```python
from build123d import *

# Parameters (mm, degrees)
SKETCH1_R           = 35
BOSS_EXTRUDE2_DEPTH = 10
SKETCH2_R           = 31
CUT_EXTRUDE1_DEPTH  = 5
SKETCH3_R           = 1.5
BOSS_EXTRUDE3_DEPTH = 5


with BuildPart() as part:
    # Sketch1 → Boss-Extrude2 (new body)
    with BuildSketch(Plane(origin=(0, 0, 0), x_dir=(1, 0, 0), z_dir=(0, 1, 0))):
        Circle(SKETCH1_R)
    extrude(amount=BOSS_EXTRUDE2_DEPTH)

    # Sketch2 → Cut-Extrude1 (cut)
    with BuildSketch(Plane(origin=(0, 10, 0), x_dir=(1, 0, 0), z_dir=(0, 1, 0))):
        Circle(SKETCH2_R)
    extrude(amount=-CUT_EXTRUDE1_DEPTH, mode=Mode.SUBTRACT)

    # Sketch3 → Boss-Extrude3 (add)
    with BuildSketch(Plane.XZ):
        Circle(SKETCH3_R)
    extrude(amount=BOSS_EXTRUDE3_DEPTH)


solid = part.part
```
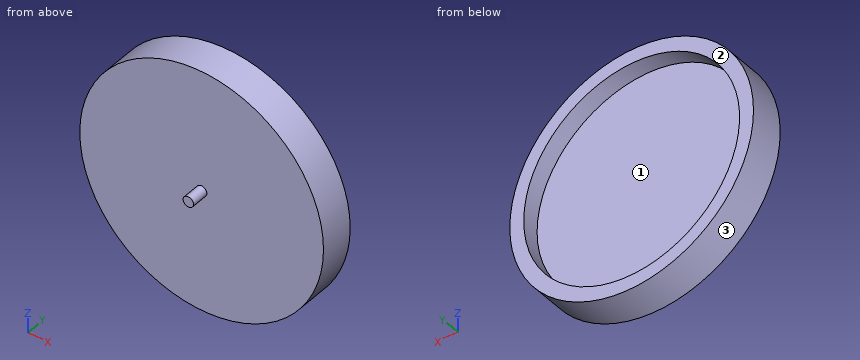
Model file for the job. Use its own axes, mm. Face numbers are marked on the shaded views. Round coordinates to 2 decimals unless told otherwise and drop trailing zeros. Write each loop counter-clockwise with the first axis right and the second up, starting at its lowest first coordinate (ties: lowest second). Pieces come first, ordered by that corner, then holes. Notation, with made-up numbers: (48.5, -24.5) - (67.5, -24.5) arc R19 cw to (67.5, 1.5) - close; hole circle Ø2 at (73.25, -22.5). An arc over 180 degrees is marked (long way). Use CSV: the item, a comma, the result in double quotes. Start each with the question number.
Item 1: Drill centre lines: L1, parallel to X at y = 6.45, z = 0; L2, parallel to Y at x = 22.5, z = -20. Where is each one in solid material? Low to high. Write a range as [from, to].
Item 2: Band-saw the part on D-D (y = -1.75). Write the cut outline in (x, z), and give its area (3 significant figures).
Item 3: Band-saw the part on C-C (y = 7.5). Write the cut outline in (x, z).
Item 4: Pin check, flat tips, straight feed: P1, Ø2, axis at x = -8, y = -0.5, coming from the -Z side; P2, Ø5, axis at x = -16.5, z = 19.5, coming from the -Y side; P3, Ø1, axis at x = -19, y = 7, coming from the +Z side. Stop position of each tip, or through.
Item 5: Two-plate mould, pull along X, no slides. Class the marked faces 1, 2 and 3: released by +X, released by -X, zero draft, split by the parting line, or undercut.
Item 6: Band-saw the part on B-B (z = 0). Write the cut outline in (x, y).
Item 7: Band-saw the part on A-A (x = 0). Write the cut outline in (y, z).
Checked values:
1,L1,"x = [-35, -31], [31, 35]"
1,L2,"y = [0, 5]"
2,outline,"circle Ø3 at (0, 0)"
2,area,"7.07 mm²"
3,outline,"circle Ø70 at (0, 0); hole circle Ø62 at (0, 0)"
4,P1,"stops at z = -34.27"
4,P2,"stops at y = 0"
4,P3,"stops at z = 29.71"
5,face 1,"undercut"
5,face 2,"zero draft"
5,face 3,"split by the parting line"
6,outline,"(-35, 0) - (-1.5, 0) - (-1.5, -5) - (1.5, -5) - (1.5, 0) - (35, 0) - (35, 10) - (31, 10) - (31, 5) - (-31, 5) - (-31, 10) - (-35, 10) - close"
7,outline,"(-5, -1.5) - (0, -1.5) - (0, -35) - (10, -35) - (10, -31) - (5, -31) - (5, 31) - (10, 31) - (10, 35) - (0, 35) - (0, 1.5) - (-5, 1.5) - close"
